from build123d import *

# Parameters (mm, degrees)
SKETCH1_W          = 100
SKETCH1_H          = 8
EXTRUDE1_DEPTH     = 200
SKETCH4_W          = 40
SKETCH4_H          = 10
EXTRUDE3_DEPTH     = 620
SKETCH5_R          = 4
CUT_EXTRUDE2_DEPTH = 620


with BuildPart() as part:
    # Sketch1 → Extrude1 (new body)
    with BuildSketch(Plane.XY):
        with Locations((7.376785714, -69.436049107)):
            Rectangle(SKETCH1_W, SKETCH1_H)
    extrude(amount=EXTRUDE1_DEPTH)

    # Sketch4 → Extrude3 (add)
    with BuildSketch(Plane(origin=(0, -65.436049107, 0), x_dir=(1, 0, 0), z_dir=(0, 1, 0))):
        with Locations((7.376785714, -195)):
            Rectangle(SKETCH4_W, SKETCH4_H)
        with Locations((7.376785714, -5)):
            Rectangle(SKETCH4_W, SKETCH4_H)
    extrude(amount=EXTRUDE3_DEPTH)

    # Sketch5 → Cut-Extrude2 (cut)
    with BuildSketch(Plane.XY.offset(200)):
        with Locations((7.376785714, 534.563950893)):
            Circle(SKETCH5_R)
    extrude(amount=-CUT_EXTRUDE2_DEPTH, mode=Mode.SUBTRACT)


solid = part.part
The model under review builds one solid part; all positions refer to its coordinate system, in mm. A direction names the side the tool comes from. Coordinates: 2 decimals unless noted, no trailing zeros. Loops run counter-clockwise (first coordinate to the right, second up) from the corner with the lowest first, then second, coordinate; pieces in that order, holes last.
(1) Wall thickness on L1, parallel to Z at x = 13, y = 83; L2, parallel to Y at x = 8, z = 153; L3, parallel to X at y = 305.5, z = 191.5: over which ranges is each line inside the solid? List them lowest first.
Determined:
L1: z = 0 to 10, 190 to 200
L2: y = -73.44 to -65.44
L3: x = -12.62 to 27.38
(2) Consider section C-C, the plane z = 19. Give the boundary of the cut face in (x, y), plus the area to 3 significant figures.
Determined:
outline: (-42.62, -73.44) - (57.38, -73.44) - (57.38, -65.44) - (-42.62, -65.44) - close
area: 800 mm2
(3) Consider section B-B, the plane x = 20.5. Give the boundary of the cut face in (y, z), plus the area to 3 significant figures.
Determined:
outline: (-73.44, 0) - (554.56, 0) - (554.56, 10) - (-65.44, 10) - (-65.44, 190) - (554.56, 190) - (554.56, 200) - (-73.44, 200) - close
area: 14,000 mm2
(4) Tool access review of faces 1 (the flat face through (7, 240, 190)), 2 (the flat face through (-12.623, 240, 195)), 3 (the flat face through (27.377, 240, 195)): name each direction out of +Z, -Z, +X, -X, +Y, -Y from which nothing blocks a thin tool from reaching the whole face with its end or side.
Determined:
face 1: +X, -X, +Y
face 2: +Z, -Z, -X, +Y
face 3: +Z, -Z, +X, +Y
(5) Consider section A-A, the plane y = 311. Give the boundary of the cut face in (x, z).
Determined:
outline: (-12.62, 0) - (27.38, 0) - (27.38, 10) - (-12.62, 10) - close; (-12.62, 190) - (27.38, 190) - (27.38, 200) - (-12.62, 200) - close
(6) Insertion check: P1, Ø8, axis at y = 311.5, z = 3.5, coming from the +X side; P2, Ø10.5, axis at x = 7.38, y = 534.56, coming from the +Z side; P3, Ø8, axis at y = 306.5, z = 3.5, coming from the -X side. Each pin has a flat end and moves straight along its axis. Give the tip position at first contact, or say it passes through.
Determined:
P1: stops at x = 27.38
P2: stops at z = 200
P3: stops at x = -12.62
(7) Draft analysis for pull direction Z (two halves, no side actions). For faces 4 (the flat face through (15, 242, 200)), 5 (the flat face through (-12.623, 240, 5)), 6 (the flat face through (7, -65.436, 99)), 7 (the flat face through (7, 240, 10)), state which applies: +Z half, -Z half, draft (parallel to the pull), parting line (faces both ways), or undercut.
Determined:
face 4: +Z half
face 5: draft
face 6: undercut
face 7: undercut
